Geometry: final body of the model. Coordinates: model frame, mm. A direction names the side the tool comes from. Give positions to 0.01 mm unless a question says otherwise; leave off trailing zeros. Loops run counter-clockwise (first coordinate to the right, second up) from the corner with the lowest first, then second, coordinate; pieces in that order, holes last. Notation, with made-up numbers: (-33.75, 42.25) -> (-24.75, 42.25) arc R25 ccw to (-24.75, 64.25) -> close; hole circle Ø5 at (-5, -18.5). An arc over 180 degrees is marked (long way). One line per item, written item: value. Start each with the question number.
from build123d import *

# Parameters (mm, degrees)
SKETCH1_R           = 1.905
SKETCH1_R_2         = 2.151722897
SKETCH1_R_3         = 3.429
BOSS_EXTRUDE1_DEPTH = 3.175
FILLET1_R           = 12.7


with BuildPart() as part:
    # Sketch1 → Boss-Extrude1 (new body)
    with BuildSketch(Plane(origin=(0, 0, 0), x_dir=(1, 0, 0), z_dir=(0, 1, 0))):
        with BuildLine():
            Line((-4.200130206, 4.7625), (-68.2625, 4.7625))
            ThreePointArc((-68.2625, 4.7625), (-73.025, 0), (-68.2625, -4.7625))
            Line((-68.2625, -4.7625), (-4.200130206, -4.7625))
            ThreePointArc((-4.200130206, -4.7625), (0, -6.35), (4.200130206, -4.7625))
            Line((4.200130206, -4.7625), (68.2625, -4.7625))
            ThreePointArc((68.2625, -4.7625), (73.025, 0), (68.2625, 4.7625))
            Line((68.2625, 4.7625), (4.200130206, 4.7625))
            ThreePointArc((4.200130206, 4.7625), (0, 6.35), (-4.200130206, 4.7625))
        make_face()
        with Locations((-68.2625, 0)):
            Circle(SKETCH1_R, mode=Mode.SUBTRACT)
        with Locations((-29.337, 0)):
            Circle(SKETCH1_R_2, mode=Mode.SUBTRACT)
        Circle(SKETCH1_R_3, mode=Mode.SUBTRACT)
        with Locations((68.2625, 0)):
            Circle(SKETCH1_R, mode=Mode.SUBTRACT)
        with Locations((29.337, 0)):
            Circle(SKETCH1_R_2, mode=Mode.SUBTRACT)
    extrude(amount=BOSS_EXTRUDE1_DEPTH)

    # Fillet1
    fillet1_edges = [part.edges().sort_by_distance(p)[0] for p in [
        (-4.200130206, 1.5875, -4.7625),
        (4.200130206, 1.5875, -4.7625),
        (4.200130206, 1.5875, 4.7625),
        (-4.200130206, 1.5875, 4.7625),
    ]]
    fillet(fillet1_edges, radius=FILLET1_R)

    # Sketch5 → Cut-Revolve2 (revolve, cut)
    with BuildSketch(Plane.XY):
        Polygon((-64.3636, 3.175), (-66.505348665, 0.7112), (-66.505348665, 3.175), align=None)
    cut_revolve2 = revolve(axis=Axis((-68.2625, 0, 0), (0, 1, 0)), mode=Mode.SUBTRACT)

    # Mirror1: Cut-Revolve2 across plane
    add(cut_revolve2.mirror(Plane(origin=(0, 0, 0), x_dir=(0, 0, 1), z_dir=(1, 0, 0))), mode=Mode.SUBTRACT)


solid = part.part
Item 1: Mould query, pull axis X, two halves, no side actions, for faces 4 (the face through (27.187, 1.565, -0.095)), 5 (the face through (38, 2, -4.762)), 6 (the face through (73.024, 1.565, 0.105)). Classes: pulls with the +X half, pulls with the -X half, needs draft (parallel to the pull), parting line crosses it, or undercut.
Item 2: Section D-D, the plane x = 28.5. Output: boundary loops of the cut face in (y, z) (1 decimal), then the cut area to 3 significant figures.
Item 3: Section A-A, the plane z = 0. Output: boundary loops of the cut face in (x, y) (1 decimal), then the cut area to 3 significant figures.
Item 4: Access query for faces 1 (the face through (-38, 2, -4.762)), 2 (the face through (38, 2, 4.762)), 3 (the face through (66.36, 0.43, -0.08)). Directions: +Z, -Z, +X, -X, +Y, -Y. A direction counts if a zero-diameter tool reaches every point of the face in a straight line with its end or side. Return the directions, or none.
Item 5: Section B-B, the plane x = 0. Output: boundary loops of the cut face in (y, z) (3 decimals), then the cut area to 3 significant figures.
Item 6: Ray query, line 1 along X through (y, z) = (0.55, 0) (1 decimal); line 2 along X through (y, z) = (1.05, -0.25); line 3 along X through (y, z) = (2.25, 2.5). Return the intervals inside material, ascending. Write a range as [from, to].
Item 7: Pin query (flat end, axial travel): pin 1 (5.5 mm diameter, centred on x = -29.337, z = 0, fed in from -Y); pin 2 (1 mm diameter, centred on x = 52, y = 2, fed in from +Z). Return the tip coordinate at first contact, or that it passes through.
Item 8: Section C-C, the plane y = 2.6. State how many separate pieces and enclosed holes the cut face has, then the cut area to 3 significant figures.
Geometry check:
1. face 4: undercut
1. face 5: needs draft
1. face 6: pulls with the +X half
2. outline: (0, -4.8) -> (3.2, -4.8) -> (3.2, -2) -> (0, -2) -> close; (0, 2) -> (3.2, 2) -> (3.2, 4.8) -> (0, 4.8) -> close
2. area: 17.7 mm2
3. outline: (-73, 0) -> (-70.2, 0) -> (-70.2, 0.9) -> (-72.2, 3.2) -> (-73, 3.2) -> close; (-66.4, 0) -> (-31.5, 0) -> (-31.5, 3.2) -> (-64.4, 3.2) -> (-66.4, 0.9) -> close; (-27.2, 0) -> (-3.4, 0) -> (-3.4, 3.2) -> (-27.2, 3.2) -> close; (3.4, 0) -> (27.2, 0) -> (27.2, 3.2) -> (3.4, 3.2) -> close; (31.5, 0) -> (66.4, 0) -> (66.4, 0.9) -> (64.4, 3.2) -> (31.5, 3.2) -> close; (70.2, 0) -> (73, 0) -> (73, 3.2) -> (72.2, 3.2) -> (70.2, 0.9) -> close
3. area: 381 mm2
4. face 1: -Z, -X, +Y, -Y
4. face 2: +Z, +X, +Y, -Y
4. face 3: +Y, -Y
5. outline: (0, -6.35) -> (3.175, -6.35) -> (3.175, -3.429) -> (0, -3.429) -> close; (0, 3.429) -> (3.175, 3.429) -> (3.175, 6.35) -> (0, 6.35) -> close
5. area: 18.5 mm2
6. line 1: x = [-73, -70.2], [-66.4, -31.5], [-27.2, -3.4], [3.4, 27.2], [31.5, 66.4], [70.2, 73]
6. line 2: x = [-73.02, -70.3], [-66.23, -31.47], [-27.2, -3.42], [3.42, 27.2], [31.47, 66.23], [70.3, 73.02]
6. line 3: x = [-72.32, -70.09], [-66.44, -2.35], [2.35, 66.44], [70.09, 72.32]
7. pin 1: stops at y = 0
7. pin 2: stops at z = 4.76
8. separate pieces: 1
8. enclosed holes: 5
8. area: 1,250 mm2
